Model file for the job. Use its own axes, mm. Face numbers are marked on the shaded views. A direction names the side the tool comes from. Coordinates: 2 decimals unless noted, no trailing zeros. Write each loop counter-clockwise with the first axis right and the second up, starting at its lowest first coordinate (ties: lowest second). Pieces come first, ordered by that corner, then holes.
Q1. Band-saw the part on A-A, the plane x = 25. Write the cut outline in (y, z), plus the area to 3 significant figures.
Q2. Pin check, flat tip, straight feed: P1, Ø8, axis at x = 34, z = 27, coming from the +Y side. Stop position of the tip, or through.
Q3. Pull direction Z, two halves, no side cores. Call the marked faces 3, 4 and 5: released by +Z, released by -Z, zero draft, split by the parting line, or undercut.
Q4. Which spindle directions (+Z, -Z, +X, -X, +Y, -Y) get a long thin tool onto all of the face, cutting with end or side? Do the marked faces 1 and 2. Say none if no direction does.
Q5. Band-saw the part on C-C, the plane y = 6.5. Write the cut outline in (x, z), plus the area to 3 significant figures.
Q6. Band-saw the part on B-B, the plane z = 23. Write the cut outline in (x, y).
Q7. Drill centre lines: probe 1 along X at (y, z) = (1.75, 1); probe 2 along Z at (x, y) = (23, 8.75). Where is each one in solid material? Low to high.
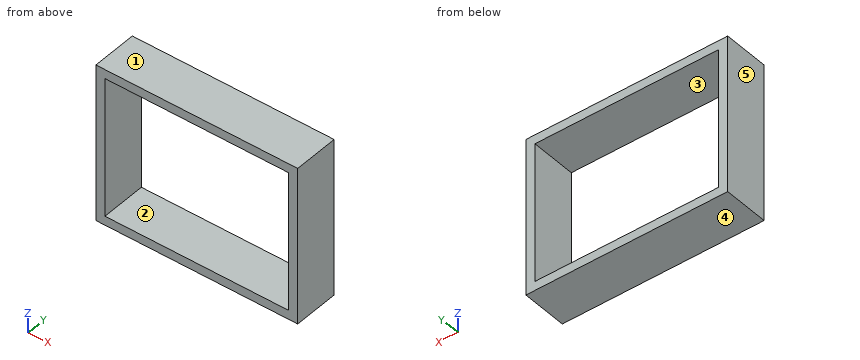
Autodesk Inventor part; units mm, degrees
ref_plane "XZ Plane" through (0, 0, 0) normal (0, 1, 0) x (-1, 0, 0)
sketch "Sketch1" plane through (0, 0, 0) normal (0, 1, 0) x (-1, 0, 0)
  line L0 (0, 0) -> (-40.5, 0)
  line L1 (-40.5, 0) -> (-40.5, 30.75)
  line L2 (-40.5, 30.75) -> (0, 30.75)
  line L3 (0, 30.75) -> (0, 0)
  line L4 (2, 32.75) -> (-42.5, 32.75)
  line L5 (-42.5, 32.75) -> (-42.5, -2)
  line L6 (-42.5, -2) -> (2, -2)
  line L7 (2, -2) -> (2, 32.75)
  dimension "d2" = 40.5
  dimension "d3" = 30.75
  dimension "d4" = 2
extrude "Extrusion1" add sketch "Sketch1" along normal blind 10
ref_plane "Work Plane19" through (0, 5, 0) normal (0, 1, 0) x (1, 0, 0)
ref_plane "Work Plane20" through (42.5, 5, 32.75) normal (-0.7071, -0.7071, 0) x (0, 0, 1)
sketch "Sketch2" plane through (42.5, 5, 32.75) normal (-0.7071, -0.7071, 0) x (0, 0, 1)
  line L0 (0, -3.5355) -> (-34.75, -3.5355) construction
  line L1 (-34.75, -3.5355) -> (-34.75, 3.5355) construction
  line L2 (0, 3.5355) -> (-34.75, 3.5355) construction
  line L3 (0, -3.5355) -> (0, 3.5355) construction
  line L4 (-41.7, 0) -> (6.95, 0) construction
  line L5 (-34.75, 0) -> (-86.722, -105.5837)
  line L6 (-32.75, 33.5876) -> (-32.75, 4.9497)
  arc A0 (-86.722, -105.5837) -> (-80.0972, -119.7206) centre (-77.75, -110) ccw construction
  line L7 (-87.75, -113.6702) -> (-87.75, -110) construction
  line L8 (-87.75, -110) -> (-87.75, -104.3872) construction
  arc A1 (-86.722, -105.5837) -> (-87.75, -110) centre (-77.75, -110) ccw
  arc A2 (-87.75, -110) -> (-84.8211, -117.0711) centre (-77.75, -110) ccw
  point P0 (-32.75, 26.5165)
  dimension "d15" = 110
  dimension "d16" = 55
  dimension "d21" = 45
  dimension "d22" = 10
properties part number "central_foot"
Answer sheet:
1. outline: (0, -2) - (10, -2) - (10, 0) - (0, 0) - close; (0, 30.75) - (10, 30.75) - (10, 32.75) - (0, 32.75) - close
1. area: 40.0 mm2
2. P1: stops at y = 10
3. face 3: undercut
3. face 4: released by -Z
3. face 5: zero draft
4. face 1: +Z, +X, -X, +Y, -Y
4. face 2: +Y, -Y
5. outline: (-2, -2) - (42.5, -2) - (42.5, 32.75) - (-2, 32.75) - close; hole (0, 0) - (40.5, 0) - (40.5, 30.75) - (0, 30.75) - close
5. area: 301 mm2
6. outline: (-2, 0) - (0, 0) - (0, 10) - (-2, 10) - close; (40.5, 0) - (42.5, 0) - (42.5, 10) - (40.5, 10) - close
7. probe 1: x = -2 to 0, 40.5 to 42.5
7. probe 2: z = -2 to 0, 30.75 to 32.75
